Read the model definition and answer for the solid it produces. Units are mm, in the model's axes. A direction names the side the tool comes from. Give positions to 0.01 mm unless a question says otherwise; leave off trailing zeros. Order: outer loops, then holes, each group sorted by start corner. A loop starts at its lowest first (then second) coordinate and runs counter-clockwise, first axis right, second up. Notation, with made-up numbers: (-37.75, 40.25) - (-4.75, 40.25) arc R19 cw to (-4.75, 62.25) - close; hole circle Ø9 at (27.5, -25.75). An arc over 180 degrees is marked (long way). Write item = value, one per line.
Autodesk Inventor part; units mm, degrees
ref_plane "YZ Plane" through (0, 0, 0) normal (1, 0, 0) x (0, 1, 0)
ref_plane "XZ Plane" through (0, 0, 0) normal (0, 1, 0) x (-1, 0, 0)
ref_plane "XY Plane" through (0, 0, 0) normal (0, 0, 1) x (1, 0, 0)
sketch "スケッチ1" plane through (0, 0, 0) normal (0, 0, 1) x (1, 0, 0)
  circle A0 centre (0, 0) radius 7.5
  circle A1 centre (0, 0) radius 12
  dimension "d0" = 15
  dimension "d1" = 24
extrude "押し出し1" add sketch "スケッチ1" along normal blind 4
sketch "スケッチ2" plane through (0, 0, 4) normal (0, 0, 1) x (1, 0, 0)
  circle A0 centre (0, 0) radius 7.5
  circle A1 centre (0, 0) radius 12
  circle A2 centre (0, 0) radius 8.5
  circle A3 centre (0, 0) radius 11
  dimension "d4" = 1
  dimension "d5" = 1
extrude "押し出し2" cut sketch "スケッチ2" against normal blind 0.5 contours A3
sketch "スケッチ3" plane through (0, 0, 0) normal (0, 0, -1) x (-1, 0, 0)
  circle A0 centre (0, 0) radius 11
  circle A1 centre (0, 0) radius 8.5
extrude "押し出し3" cut sketch "スケッチ3" against normal blind 0.5
properties part number "ベアリングd15-D24-B4" material "鋼、炭素鋼"
1. Straight lines are drawn through the part: L1, parallel to Y at x = 0, z = 3.7; L2, parallel to Y at x = 0, z = 1.25; L3, parallel to X at y = -5.75, z = 3.75. For each, find the intervals that lie inside material, in ascending order. Write a range as [from, to].
Recorded:
L1 = [-12, -11], [-8.5, -7.5], [7.5, 8.5], [11, 12]
L2 = [-12, -7.5], [7.5, 12]
L3 = [-10.53, -9.38], [-6.26, -4.82], [4.82, 6.26], [9.38, 10.53]
2. Section C-C (z = 2.9) is taken. Determine the outline of the cut face in (x, y), and give its area (3 significant figures).
Recorded:
outline = circle Ø24 at (0, 0); hole circle Ø15 at (0, 0)
area = 276 mm^2
3. For faces 4 (the face through (0, -8, 0)), 5 (the face through (2.38, -10.74, 0.25)), 6 (the face through (3.2, -8.1, 3.5)), determine the directions among +Z, -Z, +X, -X, +Y, -Y from which every point of the face is accessible in a straight line to the end or side of a thin tool.
Recorded:
face_4 = -Z, +X, -X, +Y, -Y
face_5 = -Z
face_6 = +Z
4. Flat-ended cylindrical pins translate along their axes: pin 1 (1.5 mm diameter, centred on y = -4.5, z = 1, fed in from -X); pin 2 (1 mm diameter, centred on x = -6.5, z = 2.5, fed in from -Y); pin 3 (1 mm diameter, centred on x = -6.5, z = 1.5, fed in from +Y); pin 4 (13 mm diameter, centred on x = 0, y = 0, fed in from +Z). Find the tip coordinate at first contact, or state that the pin passes through.
Recorded:
pin_1 = -11.4
pin_2 = -10.39
pin_3 = 10.39
pin_4 = through
5. Section A-A (y = 0) is taken. Determine the outline of the cut face in (x, z).
Recorded:
outline = (-12, 0) - (-11, 0) - (-11, 0.5) - (-8.5, 0.5) - (-8.5, 0) - (-7.5, 0) - (-7.5, 4) - (-8.5, 4) - (-8.5, 3.5) - (-11, 3.5) - (-11, 4) - (-12, 4) - close; (7.5, 0) - (8.5, 0) - (8.5, 0.5) - (11, 0.5) - (11, 0) - (12, 0) - (12, 4) - (11, 4) - (11, 3.5) - (8.5, 3.5) - (8.5, 4) - (7.5, 4) - close
6. Determine the mould class of faces 1 (the face through (-4.57, 7.167, 0.246)), 2 (the face through (-11.99, -0.53, 1.97)), 3 (the face through (5, -10, 0)) for opening direction Y: +Y half, -Y half, draft (parallel to the pull), parting line (faces both ways), or undercut.
Recorded:
face_1 = undercut
face_2 = parting line
face_3 = draft
7. Section D-D (x = 9.5) is taken. Determine the outline of the cut face in (y, z).
Recorded:
outline = (-7.33, 0) - (-5.55, 0) - (-5.55, 0.5) - (5.55, 0.5) - (5.55, 0) - (7.33, 0) - (7.33, 4) - (5.55, 4) - (5.55, 3.5) - (-5.55, 3.5) - (-5.55, 4) - (-7.33, 4) - close
